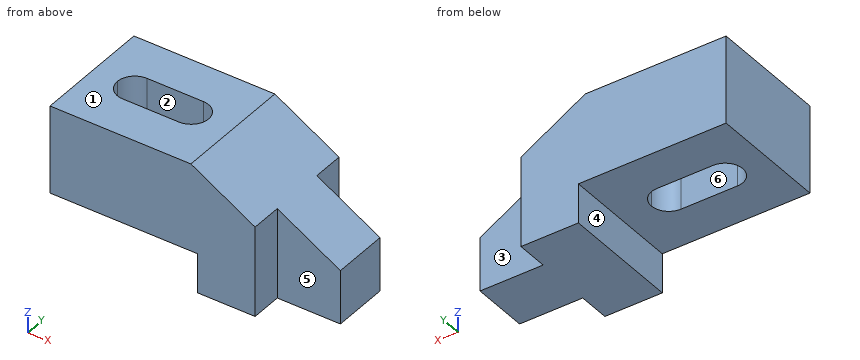
from build123d import *

# Parameters (mm, degrees)
F0_W     = 120.904
F0_H     = 57.404
F1_DEPTH = 26.924
F2_W     = 66.548
F2_H     = 17.78
F3_DEPTH = 53.849
F4_W     = 28.448
F4_H     = 14.224
F5_DEPTH = 57.405
F7_DEPTH = 57.405


with BuildPart() as f1:
    # F0 (on Front) → F1 (new body, symmetric)
    with BuildSketch(Plane.XZ):
        with Locations((60.452, 28.702)):
            Rectangle(F0_W, F0_H)
    extrude(amount=F1_DEPTH, both=True)

    # F2 (on face) → F3 (cut, through all)
    with BuildSketch(Plane.XZ.offset(26.924)):
        with Locations((33.274, 8.89)):
            Rectangle(F2_W, F2_H)
        Polygon((63.5, 57.404), (120.904, 24.2617851474), (120.904, 57.404), align=None)
    extrude(amount=-F3_DEPTH, mode=Mode.SUBTRACT)

    # F4 (on face) → F5 (cut, through all)
    with BuildSketch(Plane(origin=(0, 0, 0), x_dir=(1, 0, 0), z_dir=(0, 0, -1))):
        with Locations((106.68, 19.812)):
            Rectangle(F4_W, F4_H)
        with Locations((106.68, -19.812)):
            Rectangle(F4_W, F4_H)
    extrude(amount=-F5_DEPTH, mode=Mode.SUBTRACT)

    # F6 (on face) → F7 (cut, through all)
    with BuildSketch(Plane.XY.offset(57.404)):
        with BuildLine():
            ThreePointArc((27.178, 0), (24.8717587951, -5.5677587951), (19.304, -7.874))
            Line((19.304, -7.874), (44.704, -7.874))
            ThreePointArc((44.704, -7.874), (39.1362412049, -5.5677587951), (36.83, 0))
            Line((36.83, 0), (27.178, 0))
        make_face()
        with BuildLine():
            Line((44.704, 7.874), (19.304, 7.874))
            ThreePointArc((19.304, 7.874), (24.8717587951, 5.5677587951), (27.178, 0))
            Line((27.178, 0), (36.83, 0))
            ThreePointArc((36.83, 0), (39.1362412049, 5.5677587951), (44.704, 7.874))
        make_face()
        with BuildLine():
            ThreePointArc((19.304, 7.874), (13.7362412049, 5.5677587951), (11.43, 0))
            Line((11.43, 0), (19.304, 0))
            Line((19.304, 0), (27.178, 0))
            ThreePointArc((27.178, 0), (24.8717587951, 5.5677587951), (19.304, 7.874))
        make_face()
        with BuildLine():
            Line((19.304, 0), (11.43, 0))
            ThreePointArc((11.43, 0), (13.7362412049, -5.5677587951), (19.304, -7.874))
            ThreePointArc((19.304, -7.874), (24.8717587951, -5.5677587951), (27.178, 0))
            Line((27.178, 0), (19.304, 0))
        make_face()
        with BuildLine():
            ThreePointArc((52.578, 0), (50.2717587951, 5.5677587951), (44.704, 7.874))
            ThreePointArc((44.704, 7.874), (39.1362412049, 5.5677587951), (36.83, 0))
            ThreePointArc((36.83, 0), (39.1362412049, -5.5677587951), (44.704, -7.874))
            ThreePointArc((44.704, -7.874), (50.2717587951, -5.5677587951), (52.578, 0))
        make_face()
    extrude(amount=-F7_DEPTH, mode=Mode.SUBTRACT)


solid = f1.part
Could you check a few things on this model? Use its own coordinates, in mm. Face numbers are marked on the shaded views. A direction names the side the tool comes from. Round coordinates to 2 decimals unless told otherwise and drop trailing zeros. Order: outer loops, then holes, each group sorted by start corner. A loop starts at its lowest first (then second) coordinate and runs counter-clockwise, first axis right, second up.
(1) Imagine slicing it at D-D (z = 27). Write out the boundary of the cut face in (x, y).
Response values:
outline: (0, -26.92) - (92.46, -26.92) - (92.46, -12.7) - (116.16, -12.7) - (116.16, 12.7) - (92.46, 12.7) - (92.46, 26.92) - (0, 26.92) - close; hole (19.3, -7.87) - (44.7, -7.87) arc R7.87 ccw to (44.7, 7.87) - (19.3, 7.87) arc R7.87 ccw to start
(2) I'm going to push flat-ended pins straight in: pin 1 (15.5 mm diameter, centred on y = -21.5, z = 25.5, fed in from +X); pin 2 (4 mm diameter, centred on x = 108.5, z = 6.5, fed in from +Y); pin 3 (2 mm diameter, centred on y = 9, z = 31, fed in from +X). Where does each tip first touch, or does it pass through?
Response values:
pin 1: stops at x = 92.46
pin 2: stops at y = 12.7
pin 3: stops at x = 110.97
(3) Please list where these lines run through material, in increasing order: line 1 along X through (y, z) = (0.5, 21); line 2 along Y through (x, z) = (34.5, 37); line 3 along Z through (x, y) = (18, 14.5).
Response values:
line 1: x = 0 to 11.45, 52.56 to 120.9
line 2: y = -26.92 to -7.87, 7.87 to 26.92
line 3: z = 17.78 to 57.4
(4) Imagine slicing it at C-C (y = -19). Write out the boundary of the cut face in (x, z).
Response values:
outline: (0, 17.78) - (66.55, 17.78) - (66.55, 0) - (92.46, 0) - (92.46, 40.69) - (63.5, 57.4) - (0, 57.4) - close
(5) Imagine slicing it at A-A (z = 4). Write out the boundary of the cut face in (x, y), plus the area to 3 significant figures.
Response values:
outline: (66.55, -26.92) - (92.46, -26.92) - (92.46, -12.7) - (120.9, -12.7) - (120.9, 12.7) - (92.46, 12.7) - (92.46, 26.92) - (66.55, 26.92) - close
area: 2,120 mm2
(6) Imagine slicing it at B-B (x = 42). Write out the boundary of the cut face in (y, z), plus the area to 3 significant figures.
Response values:
outline: (-26.92, 17.78) - (-7.87, 17.78) - (-7.87, 57.4) - (-26.92, 57.4) - close; (7.87, 17.78) - (26.92, 17.78) - (26.92, 57.4) - (7.87, 57.4) - close
area: 1,510 mm2
(7) If we mould it in two halves opening along Y, with no side actions, what happens to the marked faces 1, 2 and 3? For each: released by +Y, released by -Y, zero draft, split by the parting line, or undercut.
Response values:
face 1: zero draft
face 2: undercut
face 3: released by +Y
(8) Which directions (+Z, -Z, +X, -X, +Y, -Y) give clear straight access to the entire face, cutting with the end or side of a thin tool? Please do the marked faces 4, 5 and 6.
Response values:
face 4: -Z, -X, +Y, -Y
face 5: +Z, -Z, +X, -Y
face 6: +Z, -Z
